```python
from build123d import *

# Parameters (mm, degrees)
PAD_DEPTH    = 2.6
SKETCH001_R  = 2.94
POCKET_DEPTH = 2.601
FILLET_R     = 1


with BuildPart() as part:
    # Sketch (on XY_Plane of Origin) → Pad (new body)
    with BuildSketch(Plane.XY):
        with BuildLine():
            ThreePointArc((4, -3.990301), (5.65, 0), (4, 3.990301))
            Line((4, 3.990301), (4, 8.990301))
            Line((4, 8.990301), (0, 8.990301))
            Line((0, 8.990301), (0, -5.990301))
            Line((4, -5.990301), (0, -5.990301))
            Line((4, -3.990301), (4, -5.990301))
        make_face()
    pad = extrude(amount=PAD_DEPTH)

    # Mirrored: Pad across Sketch V_Axis
    add(pad.mirror(Plane(origin=(0, 0, 0), x_dir=(0, 0, 1), z_dir=(1, 0, 0))))

    # Sketch001 (on XY_Plane of Origin) → Pocket (cut, through all)
    with BuildSketch(Plane.XY):
        Circle(SKETCH001_R)
    extrude(amount=POCKET_DEPTH, mode=Mode.SUBTRACT)

    # Fillet
    fillet_edges = [part.edges().sort_by_distance(p)[0] for p in [
        (-4, 8.990301, 1.3),
        (-4, -5.990301, 1.3),
        (4, -5.990301, 1.3),
        (4, 8.990301, 1.3),
    ]]
    fillet(fillet_edges, radius=FILLET_R)


solid = part.part
```
Here's how the part is built. I have some questions about the finished solid (model axes, mm). A direction names the side the tool comes from. Round coordinates to 2 decimals unless told otherwise and drop trailing zeros. Order: outer loops, then holes, each group sorted by start corner. A loop starts at its lowest first (then second) coordinate and runs counter-clockwise, first axis right, second up. Notation, with made-up numbers: M 39.25,29 L 65.25,29 A12 ccw 65.25,42 Z; hole C 9,61.5 d11. An arc over 180 degrees is marked long. Answer in a Markdown table with one row per item.
Item 1: Imagine slicing it at A-A, the plane x = 0. Write out the boundary of the cut face in (y, z).
A:
| item | result |
|---|---|
| outline | M -5.99,0 L -2.94,0 L -2.94,2.6 L -5.99,2.6 Z; M 2.94,0 L 8.99,0 L 8.99,2.6 L 2.94,2.6 Z |
Item 2: Imagine slicing it at B-B, the plane y = 0. Write out the boundary of the cut face in (x, z), and give its area (3 significant figures).
A:
| item | result |
|---|---|
| outline | M -5.65,0 L -2.94,0 L -2.94,2.6 L -5.65,2.6 Z; M 2.94,0 L 5.65,0 L 5.65,2.6 L 2.94,2.6 Z |
| area | 14.1 mm2 |
Item 3: If I drill on L1, parallel to X at y = 0, z = 0.95; L2, parallel to Y at x = 0, z = 1.8; L3, parallel to X at y = 7.75, z = 0.5, over which ranges is the centre line in solid material (lowest first)? Write a range as from..to.
A:
| item | result |
|---|---|
| L1 | x = -5.65..-2.94, 2.94..5.65 |
| L2 | y = -5.99..-2.94, 2.94..8.99 |
| L3 | x = -4..4 |
Item 4: For faces 1 (the face through (3.699, -5.705, 1.318)), 2 (the face through (-4, 6, 1)), 3 (the face through (4, 6, 1)), 4 (the face through (-4, -4.5, 1.3)), 5 (the face through (0, 8.99, 1)), which set-ups out of +Z, -Z, +X, -X, +Y, -Y let a thin tool reach every point of the face, with its end or its side?
A:
| item | result |
|---|---|
| face 1 | +Z, -Z, +X, -Y |
| face 2 | +Z, -Z, -X, +Y |
| face 3 | +Z, -Z, +X, +Y |
| face 4 | +Z, -Z, -X, -Y |
| face 5 | +Z, -Z, +X, -X, +Y |
Item 5: Imagine slicing it at D-D, the plane y = 5.5. Write out the boundary of the cut face in (x, z).
A:
| item | result |
|---|---|
| outline | M -4,0 L 4,0 L 4,2.6 L -4,2.6 Z |
Item 6: I'm going to push flat-ended pins straight in: pin 1 (0.5 mm diameter, centred on y = -4.5, z = 0.5, fed in from +X); pin 2 (1.5 mm diameter, centred on y = -3, z = 2, fed in from +X). Where does each tip first touch, or does it pass through?
A:
| item | result |
|---|---|
| pin 1 | stops at x = 4 |
| pin 2 | stops at x = 5.18 |
Item 7: Thinking about a two-plate mould opening in Y: for faces 6 (the face through (2.8, 0.9, 1.3)), 7 (the face through (0, -5.99, 1)), 8 (the face through (4, -4.5, 1.3)), which applies, +Y half, -Y half, draft (parallel to the pull), parting line (faces both ways), or undercut?
A:
| item | result |
|---|---|
| face 6 | undercut |
| face 7 | -Y half |
| face 8 | draft |
Item 8: Imagine slicing it at C-C, the plane z = 1. Write out the boundary of the cut face in (x, y).
A:
| item | result |
|---|---|
| outline | M -4,-4.99 A1 ccw -3,-5.99 L 3,-5.99 A1 ccw 4,-4.99 L 4,-3.99 A5.65 ccw 4,3.99 L 4,7.99 A1 ccw 3,8.99 L -3,8.99 A1 ccw -4,7.99 L -4,3.99 A5.65 ccw -4,-3.99 Z; hole C 0,0 d5.88 |
